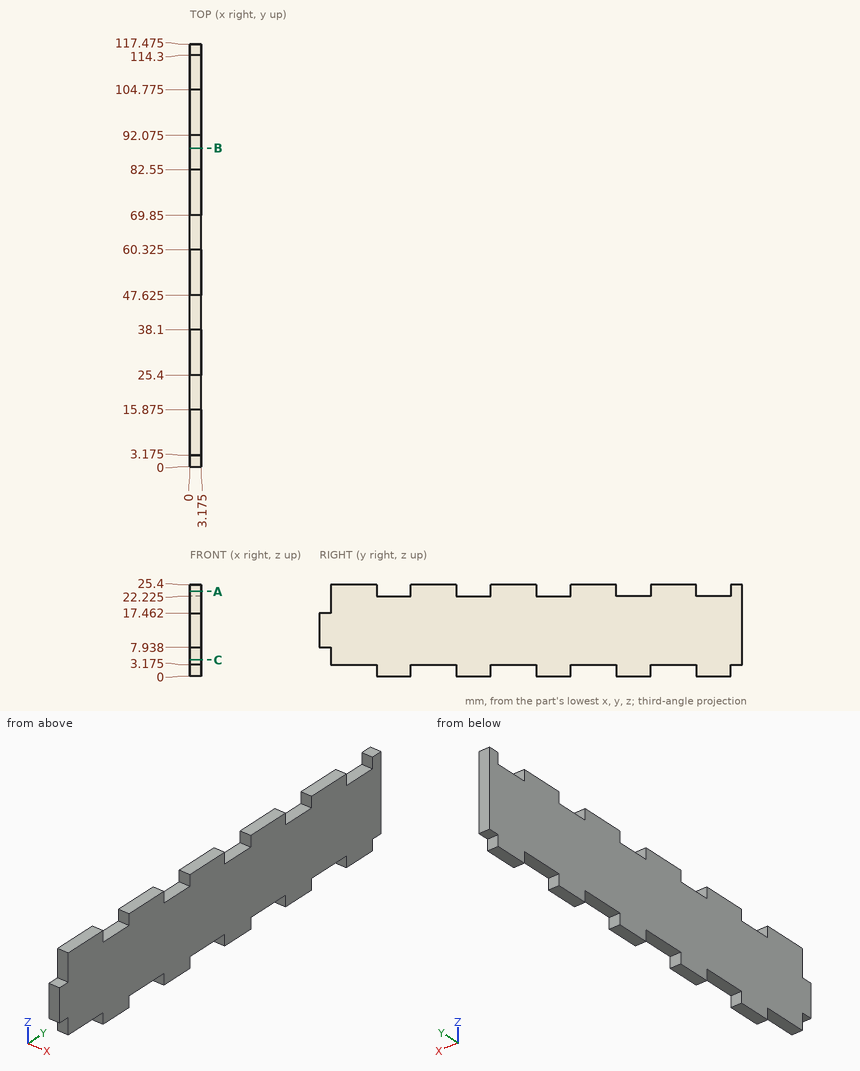
Study the drawing (mm; zero at the part's minimum x, y, z) and answer. Give positions to 0.01 mm unless a question says otherwise; leave off trailing zeros. Loops run counter-clockwise (first coordinate to the right, second up) from the corner with the lowest first, then second, coordinate; pieces in that order, holes last. Notation, with made-up numbers: (-15, 76.5) - (7, 76.5) arc R10 cw to (7, 90.5) - close; hole circle Ø5 at (35.25, -34.75). An arc over 180 degrees is marked (long way). Return JSON: item names as keys, results as strings. Group by question number.
1. Find section A-A (z = 23.5). State how many separate pieces and enclosed holes the cut face has, then the cut area to 3 significant figures.
2. Straight lines are drawn through the part: line 1 (Y direction, x = 0.6, z = 4.5) (1 decimal); line 2 (Z direction, x = 1.3, y = 46) (1 decimal); line 3 (Z direction, x = 1.9, y = 36.5) (1 decimal). For each, find the intervals that lie inside material, in ascending order. Write a range as [from, to].
3. Find section B-B (y = 88.5). Write down the section's boundary in (x, z) (1 decimal).
4. Given pin 1 Ø1 at (x, y) = (1.5, 110) entering from +Z (1 decimal); pin 2 Ø1 at (x, z) = (1.5, 23.5) entering from -Y (1 decimal); pin 3 Ø1 at (x, z) = (2.5, 1.5) entering from +Y, each flat-ended and moving along its own axis, determine where each tip first touches the part or whether it passes through.
5. Find section C-C (z = 4.5). Write down the section's boundary in (x, y) (1 decimal).
Verdict:
{
 "1": {"separate pieces": "6", "enclosed holes": "0", "area": "212 mm^2"},
 "2": {"line 1": "y = [3.2, 117.5]", "line 2": "z = [0, 22.2]", "line 3": "z = [3.2, 25.4]"},
 "3": {"outline": "(0, 0) - (3.2, 0) - (3.2, 22.2) - (0, 22.2) - close"},
 "4": {"pin 1": "stops at z = 22.2", "pin 2": "stops at y = 3.2", "pin 3": "stops at y = 114.3"},
 "5": {"outline": "(0, 3.2) - (3.2, 3.2) - (3.2, 117.5) - (0, 117.5) - close"}
}
